from build123d import *

# Parameters (mm, degrees)
F0_R     = 44.45
F0_R_2   = 6.35
F1_DEPTH = 12.7


with BuildPart() as f1:
    # F0 (on Top) → F1 (new body)
    with BuildSketch(Plane.XY):
        Circle(F0_R)
        with BuildLine():
            ThreePointArc((-4.040909, -12.039977), (-3.413958, -12.502455), (-3.175, -13.243975))
            Line((-3.175, -13.243975), (-3.175, -30.28757))
            ThreePointArc((-3.175, -30.28757), (-5.768289, -35.407103), (-11.43, -36.345084))
            ThreePointArc((-11.43, -36.345084), (-14.580239, -35.19981), (-17.617625, -33.782086))
            ThreePointArc((-17.617625, -33.782086), (-20.957806, -29.115399), (-19.171482, -23.66161))
            Line((-19.171482, -23.66161), (-7.119841, -11.609969))
            ThreePointArc((-7.119841, -11.609969), (-6.426538, -11.254603), (-5.656195, -11.370904))
            ThreePointArc((-5.656195, -11.370904), (-4.86008, -11.73327), (-4.040909, -12.039977))
        make_face(mode=Mode.SUBTRACT)
        with BuildLine():
            Line((-30.28757, -3.175), (-13.243975, -3.175))
            ThreePointArc((-13.243975, -3.175), (-12.502455, -3.413958), (-12.039977, -4.040909))
            ThreePointArc((-12.039977, -4.040909), (-11.73327, -4.86008), (-11.370904, -5.656195))
            ThreePointArc((-11.370904, -5.656195), (-11.254603, -6.426538), (-11.609969, -7.119841))
            Line((-11.609969, -7.119841), (-23.66161, -19.171482))
            ThreePointArc((-23.66161, -19.171482), (-29.115399, -20.957806), (-33.782086, -17.617625))
            ThreePointArc((-33.782086, -17.617625), (-35.19981, -14.580239), (-36.345084, -11.43))
            ThreePointArc((-36.345084, -11.43), (-35.407103, -5.768289), (-30.28757, -3.175))
        make_face(mode=Mode.SUBTRACT)
        with BuildLine():
            Line((3.175, -30.28757), (3.175, -13.243975))
            ThreePointArc((3.175, -13.243975), (3.413958, -12.502455), (4.040909, -12.039977))
            ThreePointArc((4.040909, -12.039977), (4.86008, -11.73327), (5.656195, -11.370904))
            ThreePointArc((5.656195, -11.370904), (6.426538, -11.254603), (7.119841, -11.609969))
            Line((7.119841, -11.609969), (19.171482, -23.66161))
            ThreePointArc((19.171482, -23.66161), (20.957806, -29.115399), (17.617625, -33.782086))
            ThreePointArc((17.617625, -33.782086), (14.580239, -35.19981), (11.43, -36.345084))
            ThreePointArc((11.43, -36.345084), (5.768289, -35.407103), (3.175, -30.28757))
        make_face(mode=Mode.SUBTRACT)
        with BuildLine():
            ThreePointArc((12.039977, -4.040909), (12.502455, -3.413958), (13.243975, -3.175))
            Line((13.243975, -3.175), (30.28757, -3.175))
            ThreePointArc((30.28757, -3.175), (35.407103, -5.768289), (36.345084, -11.43))
            ThreePointArc((36.345084, -11.43), (35.19981, -14.580239), (33.782086, -17.617625))
            ThreePointArc((33.782086, -17.617625), (29.115399, -20.957806), (23.66161, -19.171482))
            Line((23.66161, -19.171482), (11.609969, -7.119841))
            ThreePointArc((11.609969, -7.119841), (11.254603, -6.426538), (11.370904, -5.656195))
            ThreePointArc((11.370904, -5.656195), (11.73327, -4.86008), (12.039977, -4.040909))
        make_face(mode=Mode.SUBTRACT)
        with BuildLine():
            ThreePointArc((-12.039977, 4.040909), (-12.502455, 3.413958), (-13.243975, 3.175))
            Line((-13.243975, 3.175), (-30.28757, 3.175))
            ThreePointArc((-30.28757, 3.175), (-35.407103, 5.768289), (-36.345084, 11.43))
            ThreePointArc((-36.345084, 11.43), (-35.19981, 14.580239), (-33.782086, 17.617625))
            ThreePointArc((-33.782086, 17.617625), (-29.115399, 20.957806), (-23.66161, 19.171482))
            Line((-23.66161, 19.171482), (-11.609969, 7.119841))
            ThreePointArc((-11.609969, 7.119841), (-11.254603, 6.426538), (-11.370904, 5.656195))
            ThreePointArc((-11.370904, 5.656195), (-11.73327, 4.86008), (-12.039977, 4.040909))
        make_face(mode=Mode.SUBTRACT)
        with BuildLine():
            ThreePointArc((-17.617625, 33.782086), (-14.580239, 35.19981), (-11.43, 36.345084))
            ThreePointArc((-11.43, 36.345084), (-5.768289, 35.407103), (-3.175, 30.28757))
            Line((-3.175, 30.28757), (-3.175, 13.243975))
            ThreePointArc((-3.175, 13.243975), (-3.413958, 12.502455), (-4.040909, 12.039977))
            ThreePointArc((-4.040909, 12.039977), (-4.86008, 11.73327), (-5.656195, 11.370904))
            ThreePointArc((-5.656195, 11.370904), (-6.426538, 11.254603), (-7.119841, 11.609969))
            Line((-7.119841, 11.609969), (-19.171482, 23.66161))
            ThreePointArc((-19.171482, 23.66161), (-20.957806, 29.115399), (-17.617625, 33.782086))
        make_face(mode=Mode.SUBTRACT)
        Circle(F0_R_2, mode=Mode.SUBTRACT)
        with BuildLine():
            ThreePointArc((13.243975, 3.175), (12.502455, 3.413958), (12.039977, 4.040909))
            ThreePointArc((12.039977, 4.040909), (11.73327, 4.86008), (11.370904, 5.656195))
            ThreePointArc((11.370904, 5.656195), (11.254603, 6.426538), (11.609969, 7.119841))
            Line((11.609969, 7.119841), (23.66161, 19.171482))
            ThreePointArc((23.66161, 19.171482), (29.115399, 20.957806), (33.782086, 17.617625))
            ThreePointArc((33.782086, 17.617625), (35.19981, 14.580239), (36.345084, 11.43))
            ThreePointArc((36.345084, 11.43), (35.407103, 5.768289), (30.28757, 3.175))
            Line((30.28757, 3.175), (13.243975, 3.175))
        make_face(mode=Mode.SUBTRACT)
        with BuildLine():
            Line((3.175, 13.243975), (3.175, 30.28757))
            ThreePointArc((3.175, 30.28757), (5.768289, 35.407103), (11.43, 36.345084))
            ThreePointArc((11.43, 36.345084), (14.580239, 35.19981), (17.617625, 33.782086))
            ThreePointArc((17.617625, 33.782086), (20.957806, 29.115399), (19.171482, 23.66161))
            Line((19.171482, 23.66161), (7.119841, 11.609969))
            ThreePointArc((7.119841, 11.609969), (6.426538, 11.254603), (5.656195, 11.370904))
            ThreePointArc((5.656195, 11.370904), (4.86008, 11.73327), (4.040909, 12.039977))
            ThreePointArc((4.040909, 12.039977), (3.413958, 12.502455), (3.175, 13.243975))
        make_face(mode=Mode.SUBTRACT)
    extrude(amount=F1_DEPTH)


solid = f1.part
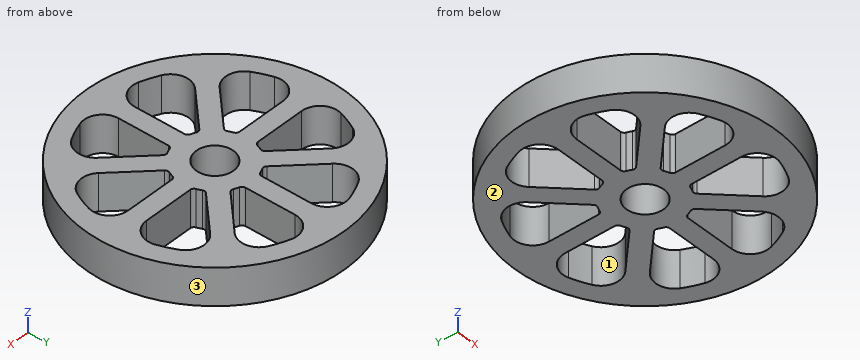
Source: CAD feature listing. Evaluate the final solid. Frame: model axes, mm. Face numbers are marked on the shaded views. Round coordinates to 2 decimals unless told otherwise and drop trailing zeros. Loops run counter-clockwise (first coordinate to the right, second up) from the corner with the lowest first, then second, coordinate; pieces in that order, holes last. Notation, with made-up numbers: (-30.5, 17) -> (-24.5, 17) arc R25 ccw to (-24.5, 50) -> close; hole circle Ø5 at (68, 88). An arc over 180 degrees is marked (long way). Answer as a JSON object with one key per item and string values. Group by question number.
Q1. Contact query for flat-ended pins moving along their axis: P1, Ø6.5, axis at y = -21.5, z = 8, coming from the -X side; P2, Ø4, axis at y = 23, z = 8, coming from the -X side; P3, Ø10, axis at x = 19.5, y = -32, coming from the +Z side; P4, Ø4, axis at x = 24.5, z = 4, coming from the +Y side. Output: stop coordinate, or through.
Q2. Section query C-C (x = 32). Output: boundary loops of the cut face in (y, z).
Q3. Mould query, pull axis X, two halves, no side actions, for the marked faces 1, 2 and 3. Classes: pulls with the +X half, pulls with the -X half, needs draft (parallel to the pull), parting line crosses it, or undercut.
Q4. Section query D-D (z = 3.75). State how many separate pieces and enclosed holes the cut face has, plus the area to 3 significant figures.
Q5. Section query A-A (x = 0). Output: boundary loops of the cut face in (y, z).
Q6. Ray query, line 1 (Y direction, x = 0, z = 4); line 2 (Y direction, x = 11.5, z = 3); line 3 (Y direction, x = -4, z = 6). Return the intervals inside material, ascending. Write a range as from..to.
Completed:
{
 "1": {"P1": "x = -40.53", "P2": "x = -39.18", "P3": "z = 12.7", "P4": "y = 38.33"},
 "2": {"outline": "(-30.85, 0) -> (-19.73, 0) -> (-19.73, 12.7) -> (-30.85, 12.7) -> close; (-3.41, 0) -> (3.41, 0) -> (3.41, 12.7) -> (-3.41, 12.7) -> close; (19.73, 0) -> (30.85, 0) -> (30.85, 12.7) -> (19.73, 12.7) -> close"},
 "3": {"face 1": "undercut", "face 2": "needs draft", "face 3": "parting line crosses it"},
 "4": {"separate pieces": "1", "enclosed holes": "9", "area": "3,560 mm²"},
 "5": {"outline": "(-44.45, 0) -> (-6.35, 0) -> (-6.35, 12.7) -> (-44.45, 12.7) -> close; (6.35, 0) -> (44.45, 0) -> (44.45, 12.7) -> (6.35, 12.7) -> close"},
 "6": {"line 1": "-44.45..-6.35, 6.35..44.45", "line 2": "-42.94..-36.32, -15.99..-6.99, -5.39..5.39, 6.99..15.99, 36.32..42.94", "line 3": "-44.27..-33.42, -12.05..-4.93, 4.93..12.05, 33.42..44.27"}
}
